from build123d import *

# Parameters (mm, degrees)
PAD_DEPTH    = 8
SKETCH001_W  = 7
SKETCH001_H  = 5
PAD001_DEPTH = 5
SKETCH002_W  = 3
SKETCH002_H  = 1.6
PAD002_DEPTH = 5
SKETCH003_W  = 7
SKETCH003_H  = 1.2
POCKET_DEPTH = 13.001


with BuildPart() as part:
    # Sketch → Pad (new body)
    with BuildSketch(Plane.XY):
        Polygon((-3.5, 2), (-3.25, 3), (-2.75, 3), (-2.5, 2), (-1.5, 2), (-1.25, 3), (-0.75, 3), (-0.5, 2), (0.5, 2), (0.75, 3), (1.25, 3), (1.5, 2), (2.5, 2), (2.75, 3), (3.25, 3), (3.5, 2), (3.5, -2), (-3.5, -2), align=None)
    extrude(amount=PAD_DEPTH)

    # Sketch001 → Pad001 (new body)
    with BuildSketch(Plane(origin=(0, 0, 0), x_dir=(1, 0, 0), z_dir=(0, 0, -1))):
        with Locations((0, -0.5)):
            Rectangle(SKETCH001_W, SKETCH001_H)
    extrude(amount=PAD001_DEPTH)

    # Sketch002 → Pad002 (new body)
    with BuildSketch(Plane.XY.offset(8)):
        Rectangle(SKETCH002_W, SKETCH002_H)
    extrude(amount=PAD002_DEPTH)

    # Sketch003 → Pocket (cut, through all)
    with BuildSketch(Plane.XY.offset(8)):
        with Locations((0, -1.4)):
            Rectangle(SKETCH003_W, SKETCH003_H)
    extrude(amount=-POCKET_DEPTH, mode=Mode.SUBTRACT)


solid = part.part
The listing builds one solid part. Answer for the finished solid, in the listing's coordinates (mm). A direction names the side the tool comes from. Coordinates: 2 decimals unless noted, no trailing zeros. Write each loop counter-clockwise with the first axis right and the second up, starting at its lowest first coordinate (ties: lowest second). Pieces come first, ordered by that corner, then holes. Notation, with made-up numbers: (-35.75, -21) - (23.25, -21) arc R19 cw to (23.25, 14) - close; hole circle Ø2 at (33, -33). An arc over 180 degrees is marked (long way). Put each result on its own line as item: value.
1. A tool of negligible diameter and unlimited length cuts with its end or side. For faces 1 (the face through (0, -0.8, 2)), 2 (the face through (0, 0.8, 10)), 3 (the face through (1.5, 0, 10)), 4 (the face through (-1.377, 2.493, 3.944)), from which of +Z, -Z, +X, -X, +Y, -Y can it reach the whole face along a straight path? Write none if from no direction.
Answer sheet:
face 1: +Z, -Z, +X, -X, -Y
face 2: +Z, +X, -X, +Y
face 3: +Z, +X, +Y, -Y
face 4: +Z, +Y
2. The part is cut by section D-D on y = 2.7. Give the vertices of the cut face in (x, z) (3 decimals).
Answer sheet:
outline: (-3.5, -5) - (3.5, -5) - (3.5, 0) - (3.325, 0) - (3.325, 8) - (2.675, 8) - (2.675, 0) - (1.325, 0) - (1.325, 8) - (0.675, 8) - (0.675, 0) - (-0.675, 0) - (-0.675, 8) - (-1.325, 8) - (-1.325, 0) - (-2.675, 0) - (-2.675, 8) - (-3.325, 8) - (-3.325, 0) - (-3.5, 0) - close
3. The part is cut by section C-C on x = 2.25. Give the vertices of the cut face in (y, z).
Answer sheet:
outline: (-0.8, -5) - (3, -5) - (3, 0) - (2, 0) - (2, 8) - (-0.8, 8) - close
4. Find the intervals of material crossed by line 1 along X through (y, z) = (2.1, 1.5) (3 decimals); line 2 along X through (y, z) = (2.6, 2.5); line 3 along Z through (x, y) = (3, 1.8), in increasing order. Write a range as from..to.
Answer sheet:
line 1: x = -3.475..-2.525, -1.475..-0.525, 0.525..1.475, 2.525..3.475
line 2: x = -3.35..-2.65, -1.35..-0.65, 0.65..1.35, 2.65..3.35
line 3: z = -5..8
5. Determine the mould class of faces 5 (the face through (3.373, 2.507, 3.944)), 6 (the face through (0.623, 2.493, 3.944)), 7 (the face through (-3.377, 2.493, 3.944)), 8 (the face through (0, 1, 8)) for opening direction X: pulls with the +X half, pulls with the -X half, needs draft (parallel to the pull), parting line crosses it, or undercut.
Answer sheet:
face 5: pulls with the +X half
face 6: undercut
face 7: pulls with the -X half
face 8: needs draft
6. Flat-ended cylindrical pins translate along their axes: pin 1 Ø1.1 at (x, y) = (-0.5, 2.5) entering from +Z; pin 2 Ø0.8 at (x, z) = (2, 3) entering from +Y; pin 3 Ø0.5 at (y, z) = (0, 10.5) entering from +X. Find the tip coordinate at first contact, or state that the pin passes through.
Answer sheet:
pin 1: stops at z = 8
pin 2: stops at y = 2
pin 3: stops at x = 1.5
7. The part is cut by section A-A on y = -0.45. Give the vertices of the cut face in (x, z).
Answer sheet:
outline: (-3.5, -5) - (3.5, -5) - (3.5, 8) - (1.5, 8) - (1.5, 13) - (-1.5, 13) - (-1.5, 8) - (-3.5, 8) - close
8. The part is cut by section B-B on z = 6.75. Give the vertices of the cut face in (x, y).
Answer sheet:
outline: (-3.5, -0.8) - (3.5, -0.8) - (3.5, 2) - (3.25, 3) - (2.75, 3) - (2.5, 2) - (1.5, 2) - (1.25, 3) - (0.75, 3) - (0.5, 2) - (-0.5, 2) - (-0.75, 3) - (-1.25, 3) - (-1.5, 2) - (-2.5, 2) - (-2.75, 3) - (-3.25, 3) - (-3.5, 2) - close
